from build123d import *

# Parameters (mm, degrees)
BOSS_EXTRUDE1_DEPTH = 5
BOSS_EXTRUDE2_DEPTH = 16
CUT_EXTRUDE1_DEPTH  = 69.893033029
SKETCH4_R           = 2.6
CUT_EXTRUDE2_DEPTH  = 16
FILLET1_R           = 1
FILLET2_R           = 1


with BuildPart() as part:
    # Sketch1 → Boss-Extrude1 (new body)
    with BuildSketch(Plane.XY):
        with BuildLine():
            Line((-34.5, -25.1), (-34.5, -32.5))
            Line((-34.5, -32.5), (34.5, -32.5))
            Line((34.5, -32.5), (34.5, -25.1))
            Line((34.5, -25.1), (27, -25.1))
            ThreePointArc((27, -25.1), (24.4, -22.5), (27, -19.9))
            Line((27, -19.9), (34.5, -19.9))
            Line((34.5, -19.9), (34.5, -7.5))
            Line((34.5, -7.5), (22.5, -7.5))
            Line((22.5, -7.5), (22.5, 32.5))
            Line((22.5, 32.5), (-22.5, 32.5))
            Line((-22.5, 32.5), (-22.5, -7.5))
            Line((-22.5, -7.5), (-34.5, -7.5))
            Line((-34.5, -7.5), (-34.5, -19.9))
            Line((-34.5, -19.9), (-27, -19.9))
            ThreePointArc((-27, -19.9), (-24.4, -22.5), (-27, -25.1))
            Line((-27, -25.1), (-34.5, -25.1))
        make_face()
        with BuildLine():
            ThreePointArc((-14, 15.5), (-12, 17.5), (-10, 15.5))
            Line((-10, 15.5), (-10, 13.5))
            ThreePointArc((-10, 13.5), (-12, 11.5), (-14, 13.5))
            Line((-14, 13.5), (-14, 15.5))
        make_face(mode=Mode.SUBTRACT)
        with BuildLine():
            ThreePointArc((-2, 27.5), (0, 29.5), (2, 27.5))
            Line((2, 27.5), (2, 23.761355821))
            ThreePointArc((2, 23.761355821), (6.680194608, 20.75594901), (8.5, 15.5))
            Line((8.5, 15.5), (8.5, 13.5))
            ThreePointArc((8.5, 13.5), (6.680194608, 8.24405099), (2, 5.238644179))
            Line((2, 5.238644179), (2, 1.5))
            ThreePointArc((2, 1.5), (0, -0.5), (-2, 1.5))
            Line((-2, 1.5), (-2, 5.238644179))
            ThreePointArc((-2, 5.238644179), (-6.680194608, 8.24405099), (-8.5, 13.5))
            Line((-8.5, 13.5), (-8.5, 15.5))
            ThreePointArc((-8.5, 15.5), (-6.680194608, 20.75594901), (-2, 23.761355821))
            Line((-2, 23.761355821), (-2, 27.5))
        make_face(mode=Mode.SUBTRACT)
        with BuildLine():
            Line((10, 13.5), (10, 15.5))
            ThreePointArc((10, 15.5), (12, 17.5), (14, 15.5))
            Line((14, 15.5), (14, 13.5))
            ThreePointArc((14, 13.5), (12, 11.5), (10, 13.5))
        make_face(mode=Mode.SUBTRACT)
    extrude(amount=BOSS_EXTRUDE1_DEPTH)

    # Sketch2 → Boss-Extrude2 (add)
    with BuildSketch(Plane.XY.offset(5)):
        Polygon((-22.5, 32.5), (-17.5, 32.5), (-17.5, -7.5), (17.5, -7.5), (17.5, 32.5), (22.5, 32.5), (22.5, -7.5), (34.5, -7.5), (34.5, -12.5), (-34.5, -12.5), (-34.5, -7.5), (-22.5, -7.5), align=None)
    extrude(amount=BOSS_EXTRUDE2_DEPTH)

    # Sketch3 → Cut-Extrude1 (cut, through all)
    with BuildSketch(Plane(origin=(22.5, 0, 0), x_dir=(0, 0, -1), z_dir=(1, 0, 0))):
        Polygon((-21, -7.5), (-21, 32.5), (-5, 32.5), align=None)
    extrude(amount=-CUT_EXTRUDE1_DEPTH, mode=Mode.SUBTRACT)

    # Sketch4 → Cut-Extrude2 (cut)
    with BuildSketch(Plane.XZ.offset(12.5)):
        with Locations((-28.5, 15)):
            Circle(SKETCH4_R)
        with Locations(Location((28.5, 15, 0), (0, 0, 90))):
            Circle(SKETCH4_R)
    extrude(amount=-CUT_EXTRUDE2_DEPTH, mode=Mode.SUBTRACT)

    # Fillet1
    fillet1_edges = [part.edges().sort_by_distance(p)[0] for p in [
        (-34.5, -12.5, 13),
        (34.5, -12.5, 13),
        (-22.5, 32.5, 2.5),
        (22.5, 32.5, 2.5),
        (34.5, -32.5, 2.5),
        (-34.5, -32.5, 2.5),
        (-34.5, -7.5, 10.5),
        (34.5, -7.5, 10.5),
    ]]
    fillet(fillet1_edges, radius=FILLET1_R)

    # Fillet2
    fillet2_edges = [part.edges().sort_by_distance(p)[0] for p in [
        (-2, 5.238644179, 2.5),
        (2, 5.238644179, 2.5),
        (2, 23.761355821, 2.5),
        (-2, 23.761355821, 2.5),
    ]]
    fillet(fillet2_edges, radius=FILLET2_R)


solid = part.part
Read the model definition and answer for the solid it produces. Units are mm, in the model's axes. A direction names the side the tool comes from. Give positions to 0.01 mm unless a question says otherwise; leave off trailing zeros. Write each loop counter-clockwise with the first axis right and the second up, starting at its lowest first coordinate (ties: lowest second). Pieces come first, ordered by that corner, then holes. Notation, with made-up numbers: (84, -9) -> (92, -9) arc R20 ccw to (92, 12) -> close; hole circle Ø6 at (-14, -17). An arc over 180 degrees is marked (long way). Answer as a JSON object with one key per item and string values. Group by question number.
1) Consider L1, parallel to Z at x = 28.5, y = -9.6; L2, parallel to X at y = 13, z = 1.25; L3, parallel to Y at x = -12, z = 9. Determine where each line is inside the solid, lowest interval first. Write a range as from..to.
2) Each of these flat-tipped pins is pushed along its axis until it touches: P1, Ø1.6, axis at y = 15, z = 3, coming from the -X side; P2, Ø1.6, axis at y = 15, z = 2.5, coming from the +X side; P3, Ø2, axis at y = -23.5, z = 5.5, coming from the +X side. Where does it stop, or does it pass through?
3) Find section D-D (z = 8). Write down the section's boundary in (x, y), and give its area (3 significant figures).
4) Find section A-A (x = -12). Write down the section's boundary in (y, z).
5) A tool of negligible diameter and unlimited length cuts with its end or side. For faces 4 (the flat face through (34.5, -28, 2)), 5 (the flat face through (31, -19.9, 2)), 6 (the cylindrical face through (-6.85, 8.47, 2.46)), 7 (the flat face through (28, -7.5, 10)), from which of +Z, -Z, +X, -X, +Y, -Y can it reach the whole face along a straight path? Write none if from no direction.
6) Find section B-B (x = -28.5). Write down the section's boundary in (y, z), and give its area (3 significant figures).
7) The mould has two halves that part along Z. Classify faces 1 (the cylindrical face through (-30.563, -10.035, 13.418)), 2 (the flat face through (-34.5, -10, 6)), 3 (the flat face through (0, -22, 5)): +Z half, -Z half, draft (parallel to the pull), parting line (faces both ways), or undercut.
8) Find section C-C (z = 15). Write down the section's boundary in (x, y).
Values follow:
{
 "1": {"L1": "z = 0..12.4, 17.6..21", "L2": "x = -22.5..-13.94, -10.06..-8.49, 8.49..10.06, 13.94..22.5", "L3": "y = -12.5..-7.5"},
 "2": {"P1": "stops at x = -22.5", "P2": "stops at x = 22.5", "P3": "stops at x = 25.19"},
 "3": {"outline": "(-34.5, -11.5) arc R1 ccw to (-33.5, -12.5) -> (33.5, -12.5) arc R1 ccw to (34.5, -11.5) -> (34.5, -8.5) arc R1 ccw to (33.5, -7.5) -> (22.5, -7.5) -> (22.5, 25) -> (17.5, 25) -> (17.5, -7.5) -> (-17.5, -7.5) -> (-17.5, 25) -> (-22.5, 25) -> (-22.5, -7.5) -> (-33.5, -7.5) arc R1 ccw to (-34.5, -8.5) -> close", "area": "669 mm2"},
 "4": {"outline": "(-32.5, 0) -> (11.5, 0) -> (11.5, 5) -> (-7.5, 5) -> (-7.5, 21) -> (-12.5, 21) -> (-12.5, 5) -> (-32.5, 5) -> close; (17.5, 0) -> (32.5, 0) -> (32.5, 5) -> (17.5, 5) -> close"},
 "5": {"face 4": "+Z, -Z, +X, +Y, -Y", "face 5": "+Z, -Z, +X", "face 6": "+Z, -Z", "face 7": "+Z, -Z, +X, +Y"},
 "6": {"outline": "(-32.5, 0) -> (-25.1, 0) -> (-25.1, 5) -> (-32.5, 5) -> close; (-19.9, 0) -> (-7.5, 0) -> (-7.5, 12.4) -> (-12.5, 12.4) -> (-12.5, 5) -> (-19.9, 5) -> close; (-12.5, 17.6) -> (-7.5, 17.6) -> (-7.5, 21) -> (-12.5, 21) -> close", "area": "153 mm2"},
 "7": {"face 1": "undercut", "face 2": "draft", "face 3": "+Z half"},
 "8": {"outline": "(-34.5, -11.5) arc R1 ccw to (-33.5, -12.5) -> (-31.1, -12.5) -> (-31.1, -7.5) -> (-33.5, -7.5) arc R1 ccw to (-34.5, -8.5) -> close; (-25.9, -12.5) -> (25.9, -12.5) -> (25.9, -7.5) -> (22.5, -7.5) -> (22.5, 7.5) -> (17.5, 7.5) -> (17.5, -7.5) -> (-17.5, -7.5) -> (-17.5, 7.5) -> (-22.5, 7.5) -> (-22.5, -7.5) -> (-25.9, -7.5) -> close; (31.1, -12.5) -> (33.5, -12.5) arc R1 ccw to (34.5, -11.5) -> (34.5, -8.5) arc R1 ccw to (33.5, -7.5) -> (31.1, -7.5) -> close"}
}
